Geometry check sheet. Reference: the model listing, model coordinates, mm. Face numbers are marked on the shaded views. A direction names the side the tool comes from. Round coordinates to 2 decimals unless told otherwise and drop trailing zeros. Order: outer loops, then holes, each group sorted by start corner. A loop starts at its lowest first (then second) coordinate and runs counter-clockwise, first axis right, second up. Notation, with made-up numbers: (-25.75, 34) -> (28.25, 34) arc R10 ccw to (28.25, 40) -> close; hole circle Ø6 at (-8, 29). An arc over 180 degrees is marked (long way). Use a Markdown table: item, result. Add a question column.
Item 1: Gauge pin test, flat ends, axial feed: pin 1 Ø3 at (x, z) = (-8.5, 0.5) entering from -Y; pin 2 Ø6 at (x, z) = (-4.5, 3) entering from -Y; pin 3 Ø6 at (y, z) = (5.5, 2) entering from -X. Record the tip position at first contact, or that the pin passes through.
Item 2: Set-up check for the marked faces 5 and 6: record each of +Z, -Z, +X, -X, +Y, -Y from which the full face is reachable in a straight line by a thin tool's end or side.
Item 3: Mould release check, pull along Z, two halves, no side actions. Record for the marked faces 1, 2, 3 and 4: pulls with the +Z half, pulls with the -Z half, needs draft (parallel to the pull), parting line crosses it, or undercut.
Item 4: Sectioned sample at C-C, the plane z = 0.5. Record the cut outline in (x, y).
Item 5: Sectioned sample at A-A, the plane x = 0. Record the cut outline in (y, z), and give its area (3 significant figures).
Item 6: Material ranges on probe 1 along Y at (x, z) = (0, -3.5); probe 2 along X at (y, z) = (1, 2.5); probe 3 along Z at (x, y) = (6, -10.5), recorded low to high. Write a range as [from, to].
Item 7: Sectioned sample at D-D, the plane z = -5. Record the cut outline in (x, y).
from build123d import *

# Parameters (mm, degrees)
SKETCH1_R           = 11.5
SKETCH1_R_2         = 6.5
BOSS_EXTRUDE1_DEPTH = 6.25
SKETCH2_R           = 14.5
SKETCH2_R_2         = 6.5
BOSS_EXTRUDE2_DEPTH = 1
CHAMFER1_SIZE       = 2.100622615
CHAMFER1_SIZE_2     = 3
CHAMFER2_SIZE       = 1
CHAMFER3_SIZE       = 0.5


with BuildPart() as part:
    # Sketch1 → Boss-Extrude1 (new, symmetric)
    with BuildSketch(Plane.XY):
        Circle(SKETCH1_R)
        Circle(SKETCH1_R_2, mode=Mode.SUBTRACT)
    extrude(amount=BOSS_EXTRUDE1_DEPTH, both=True)

    # Sketch2 → Boss-Extrude2 (add)
    with BuildSketch(Plane.XY.offset(6.25)):
        Circle(SKETCH2_R)
        Circle(SKETCH2_R_2, mode=Mode.SUBTRACT)
    boss_extrude2 = extrude(amount=BOSS_EXTRUDE2_DEPTH)

    # Mirror1: Boss-Extrude2 across plane
    add(boss_extrude2.mirror(Plane.XY))

    # Chamfer1
    # the kernel refuses this chamfer: 3, 2.100622615 mm, written as the material it adds along each edge
    with BuildSketch(Plane(origin=(0, 0, -6.25), x_dir=(1, 0, 0), z_dir=(0, -1, 0))) as chamfer1_piece_1_section:
        Polygon((11.5, CHAMFER1_SIZE), (11.5 + CHAMFER1_SIZE_2, 0), (11.5, 0), align=None)
    chamfer1_piece_1 = revolve(axis=Axis((0, 0, -6.25), (0, 0, 1)), mode=Mode.PRIVATE)
    chamfer1_piece_1 = chamfer1_piece_1 & Plane(origin=(0, 0, -5.218650002), x_dir=(1, 0, 0), z_dir=(0, 0, 1)) * Cylinder(14.5, 58, mode=Mode.PRIVATE)
    add(chamfer1_piece_1)
    with BuildSketch(Plane(origin=(0, 0, 6.25), x_dir=(1, 0, 0), z_dir=(0, -1, 0))) as chamfer1_piece_2_section:
        Polygon((11.5, -CHAMFER1_SIZE), (11.5 + CHAMFER1_SIZE_2, 0), (11.5, 0), align=None)
    chamfer1_piece_2 = revolve(axis=Axis((0, 0, 6.25), (0, 0, 1)), mode=Mode.PRIVATE)
    chamfer1_piece_2 = chamfer1_piece_2 & Plane(origin=(0, 0, 5.218650002), x_dir=(1, 0, 0), z_dir=(0, 0, -1)) * Cylinder(14.5, 58, mode=Mode.PRIVATE)
    add(chamfer1_piece_2)

    # Chamfer2
    chamfer2_edges = [part.edges().sort_by_distance(p)[0] for p in [
        (-6.5, 0, 7.25),
        (-6.5, 0, -7.25),
    ]]
    chamfer(chamfer2_edges, length=CHAMFER2_SIZE)

    # Chamfer3
    chamfer3_edges = [part.edges().sort_by_distance(p)[0] for p in [
        (-14.5, 0, 7.25),
        (-14.5, 0, -7.25),
    ]]
    chamfer(chamfer3_edges, length=CHAMFER3_SIZE)


solid = part.part
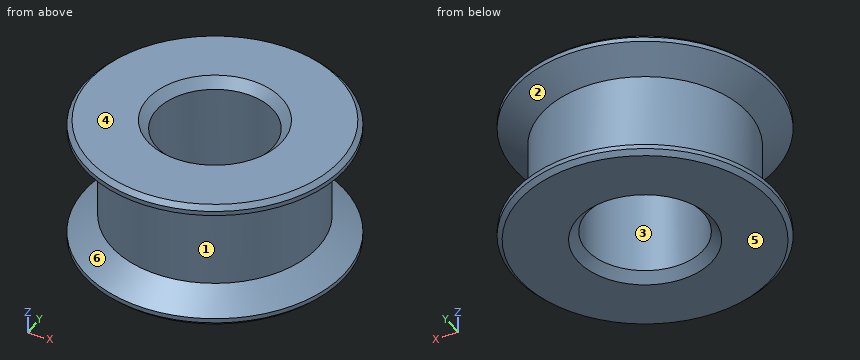
Found:
| question | item | result |
|---|---|---|
| 1 | pin 1 | stops at y = -9.12 |
| 1 | pin 2 | stops at y = -13.5 |
| 1 | pin 3 | stops at x = -11.65 |
| 2 | face 5 | -Z, +X, -X, +Y, -Y |
| 2 | face 6 | none |
| 3 | face 1 | undercut |
| 3 | face 2 | undercut |
| 3 | face 3 | needs draft |
| 3 | face 4 | pulls with the +Z half |
| 4 | outline | circle Ø23 at (0, 0); hole circle Ø13 at (0, 0) |
| 5 | outline | (-14.5, -6.75) -> (-14, -7.25) -> (-7.5, -7.25) -> (-6.5, -6.25) -> (-6.5, 6.25) -> (-7.5, 7.25) -> (-14, 7.25) -> (-14.5, 6.75) -> (-14.5, 6.25) -> (-11.5, 4.15) -> (-11.5, -4.15) -> (-14.5, -6.25) -> close; (6.5, -6.25) -> (7.5, -7.25) -> (14, -7.25) -> (14.5, -6.75) -> (14.5, -6.25) -> (11.5, -4.15) -> (11.5, 4.15) -> (14.5, 6.25) -> (14.5, 6.75) -> (14, 7.25) -> (7.5, 7.25) -> (6.5, 6.25) -> close |
| 5 | area | 167 mm2 |
| 6 | probe 1 | y = [-11.5, -6.5], [6.5, 11.5] |
| 6 | probe 2 | x = [-11.46, -6.42], [6.42, 11.46] |
| 6 | probe 3 | z = [-7.25, -4.56], [4.56, 7.25] |
| 7 | outline | circle Ø25.43 at (0, 0); hole circle Ø13 at (0, 0) |
